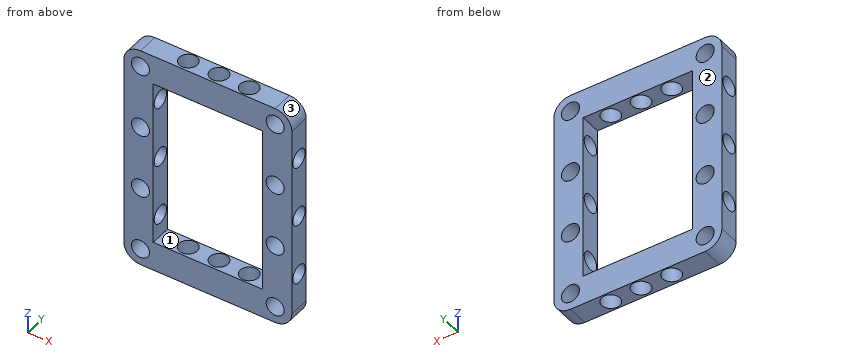
```python
from build123d import *

# Parameters (mm, degrees)
F0_W     = 26
F0_H     = 40
F1_DEPTH = 5
F2_R     = 2.15
F3_DEPTH = 5.001
F4_R     = 2.15
F5_DEPTH = 54.001
F6_R     = 2.15
F7_DEPTH = 40.001


with BuildPart() as f1:
    # F0 (on Front) → F1 (new body)
    with BuildSketch(Plane.XZ):
        with BuildLine():
            ThreePointArc((20, 23.035), (18.838678, 25.838678), (16.035, 27))
            Line((16.035, 27), (-16.035, 27))
            ThreePointArc((-16.035, 27), (-18.838678, 25.838678), (-20, 23.035))
            Line((-20, 23.035), (-20, -23.035))
            ThreePointArc((-20, -23.035), (-18.838678, -25.838678), (-16.035, -27))
            Line((-16.035, -27), (16.035, -27))
            ThreePointArc((16.035, -27), (18.838678, -25.838678), (20, -23.035))
            Line((20, -23.035), (20, 23.035))
        make_face()
        Rectangle(F0_W, F0_H, mode=Mode.SUBTRACT)
    extrude(amount=F1_DEPTH)

    # F2 (on face) → F3 (cut, through all)
    with BuildSketch(Plane.XZ.offset(5)):
        with Locations((-16.035, -23.035)):
            Circle(F2_R)
        with Locations((-16.035, -7.677)):
            Circle(F2_R)
        with Locations((-16.035, 7.679)):
            Circle(F2_R)
        with Locations((-16.035, 23.035)):
            Circle(F2_R)
        with Locations((16.035, 23.035)):
            Circle(F2_R)
        with Locations((16.035, 7.679)):
            Circle(F2_R)
        with Locations((16.035, -7.677)):
            Circle(F2_R)
        with Locations((16.035, -23.035)):
            Circle(F2_R)
    extrude(amount=-F3_DEPTH, mode=Mode.SUBTRACT)

    # F4 (on face) → F5 (cut, through all)
    with BuildSketch(Plane.XY.offset(27)):
        with Locations((8.15, -2.5)):
            Circle(F4_R)
        with Locations((0.851398, -2.357123)):
            Circle(F4_R)
        with Locations((-6.448602, -2.357123)):
            Circle(F4_R)
    extrude(amount=-F5_DEPTH, mode=Mode.SUBTRACT)

    # F6 (on face) → F7 (cut, through all)
    with BuildSketch(Plane(origin=(-20, 0, 0), x_dir=(0, -1, 0), z_dir=(-1, 0, 0))):
        with Locations((2.5, 14.575)):
            Circle(F6_R)
        with Locations((2.5, 0)):
            Circle(F6_R)
        with Locations((2.5, -14.575)):
            Circle(F6_R)
    extrude(amount=-F7_DEPTH, mode=Mode.SUBTRACT)


solid = f1.part
```
The model under review builds one solid part; all positions refer to its coordinate system, in mm. Face numbers are marked on the shaded views. Round coordinates to 2 decimals unless told otherwise and drop trailing zeros. Loops run counter-clockwise (first coordinate to the right, second up) from the corner with the lowest first, then second, coordinate; pieces in that order, holes last.
Item 1: Take a section at C-C (x = -2). Write out the cut boundary in (y, z), then the cut area to 3 significant figures.
Determined:
outline: (-5, -27) - (0, -27) - (0, -20) - (-5, -20) - close; (-5, 20) - (0, 20) - (0, 27) - (-5, 27) - close
area: 70.0 mm2
Item 2: Take a section at D-D (y = -3.9). Give the number of separate pieces and of enclosed holes in the cut face, then the cut area to 3 significant figures.
Determined:
separate pieces: 12
enclosed holes: 8
area: 724 mm2
Item 3: Clearance check with flat-ended pins moving along their axes: pin 1 Ø5.5 at (x, z) = (-16.035, -23.035) entering from -Y; pin 2 Ø3 at (x, z) = (-11, 13) entering from +Y. State where each tip first meets the part, or that it passes through.
Determined:
pin 1: stops at y = -5
pin 2: passes through
Item 4: Take a section at B-B (z = 0). Write out the cut boundary in (x, y), then the cut area to 3 significant figures.
Determined:
outline: (-20, -5) - (-13, -5) - (-13, -4.65) - (-20, -4.65) - close; (-20, -0.35) - (-13, -0.35) - (-13, 0) - (-20, 0) - close; (13, -5) - (20, -5) - (20, -4.65) - (13, -4.65) - close; (13, -0.35) - (20, -0.35) - (20, 0) - (13, 0) - close
area: 9.80 mm2
Item 5: For line 1 (X direction, y = -2.75, z = -3); line 2 (X direction, y = -2.85, z = -24); line 3 (Z direction, x = -10, y = -2.3), list the stretches that pass through material, from the lowest coordinate up.
Determined:
line 1: x = -20 to -13, 13 to 20
line 2: x = -19.88 to -17.96, -14.11 to -8.54, -4.36 to -1.24, 2.94 to 6.03, 10.27 to 14.11, 17.96 to 19.88
line 3: z = -27 to -20, 20 to 27
Item 6: Mouldability with a two-part tool opening along X and no side actions: class the marked faces 1, 2 and 3 as released by +X, released by -X, zero draft, split by the parting line, or undercut.
Determined:
face 1: undercut
face 2: zero draft
face 3: released by +X
Item 7: Take a section at A-A (x = 8.15). Write out the cut boundary in (y, z).
Determined:
outline: (-5, -27) - (-4.65, -27) - (-4.65, -20) - (-5, -20) - close; (-5, 20) - (-4.65, 20) - (-4.65, 27) - (-5, 27) - close; (-0.35, -27) - (0, -27) - (0, -20) - (-0.35, -20) - close; (-0.35, 20) - (0, 20) - (0, 27) - (-0.35, 27) - close
